Can you work these out from the model? Positions are in its coordinate system, mm. A direction names the side the tool comes from. Coordinates: 2 decimals unless noted, no trailing zeros. Order: outer loops, then holes, each group sorted by start corner. A loop starts at its lowest first (then second) coordinate and runs counter-clockwise, first axis right, second up.
```python
from build123d import *

# Parameters (mm, degrees)
SKETCH1_W           = 22.86
SKETCH1_H           = 20.32
SKETCH1_R           = 1.65
BOSS_EXTRUDE1_DEPTH = 2
SKETCH2_W           = 11.796284554
SKETCH2_H           = 1.966047426
BOSS_EXTRUDE2_DEPTH = 10
SKETCH3_W           = 7.246289084
SKETCH3_H           = 4.830859388
BOSS_EXTRUDE3_DEPTH = 8


with BuildPart() as part:
    # Sketch1 → Boss-Extrude1 (new body)
    with BuildSketch(Plane(origin=(0, 0, 0), x_dir=(1, 0, 0), z_dir=(0, 1, 0))):
        Rectangle(SKETCH1_W, SKETCH1_H)
        with Locations(Location((-8.5, 7.555555556, 0), (0, 0, 270))):
            Circle(SKETCH1_R, mode=Mode.SUBTRACT)
        with Locations(Location((8.5, 7.555555556, 0), (0, 0, 270))):
            Circle(SKETCH1_R, mode=Mode.SUBTRACT)
        with Locations(Location((-8.5, -7.555555556, 0), (0, 0, 270))):
            Circle(SKETCH1_R, mode=Mode.SUBTRACT)
        with Locations(Location((8.5, -7.555555556, 0), (0, 0, 270))):
            Circle(SKETCH1_R, mode=Mode.SUBTRACT)
    extrude(amount=BOSS_EXTRUDE1_DEPTH)

    # Sketch2 → Boss-Extrude2 (add)
    with BuildSketch(Plane.XZ):
        with Locations((0, 7.569282589)):
            Rectangle(SKETCH2_W, SKETCH2_H)
    extrude(amount=BOSS_EXTRUDE2_DEPTH)

    # Sketch3 → Boss-Extrude3 (add)
    with BuildSketch(Plane.XZ):
        with Locations((0, -7.288418671)):
            Rectangle(SKETCH3_W, SKETCH3_H)
    extrude(amount=BOSS_EXTRUDE3_DEPTH)


solid = part.part
```
1. Please list where these lines run through material, in increasing order: probe 1 along Z at (x, y) = (0, -4.5); probe 2 along Y at (x, z) = (9.75, -1.25); probe 3 along Z at (x, y) = (4.5, -2.5).
Completed:
probe 1: z = -9.7 to -4.87, 6.59 to 8.55
probe 2: y = 0 to 2
probe 3: z = 6.59 to 8.55
2. On a 3-axis mill with a long thin cutter (end or side, diameter ignored), from which of +Z, -Z, +X, -X, +Y, -Y can I reach the whole of each face in a straight line? I mean faces 1 (the flat face through (0, -5, 8.552)), 2 (the flat face through (-3.623, -4, -7)), 3 (the flat face through (0, -4, -9.704)), 4 (the flat face through (-5.898, -5, 8)), 5 (the flat face through (0, -5, 6.586)). Say none if no direction works.
Completed:
face 1: +Z, +X, -X, -Y
face 2: -Z, -X, -Y
face 3: -Z, +X, -X, -Y
face 4: +Z, -Z, -X, -Y
face 5: +X, -X, -Y
3. Imagine slicing it at A-A on x = -8.5. Please give me the cut outline in (y, z).
Completed:
outline: (0, -10.16) - (2, -10.16) - (2, -9.21) - (0, -9.21) - close; (0, -5.91) - (2, -5.91) - (2, 5.91) - (0, 5.91) - close; (0, 9.21) - (2, 9.21) - (2, 10.16) - (0, 10.16) - close
4. Thinking about a two-plate mould opening in Z: for faces 6 (the cylindrical face through (7.87, 0.99, 9.08)), 7 (the flat face through (0, 1, 10.16)), 8 (the flat face through (5.898, -5, 8)), which applies, pulls with the +Z half, pulls with the -Z half, needs draft (parallel to the pull), parting line crosses it, or undercut?
Completed:
face 6: undercut
face 7: pulls with the +Z half
face 8: needs draft
5. Imagine slicing it at B-B on y = -2. Please give me the cut outline in (x, z), then the cut area to 3 significant figures.
Completed:
outline: (-5.9, 6.59) - (5.9, 6.59) - (5.9, 8.55) - (-5.9, 8.55) - close; (-3.62, -9.7) - (3.62, -9.7) - (3.62, -4.87) - (-3.62, -4.87) - close
area: 58.2 mm2
6. Imagine slicing it at C-C on y = 1.5. Please give me the cut outline in (x, z), then the cut area to 3 significant figures.
Completed:
outline: (-11.43, -10.16) - (11.43, -10.16) - (11.43, 10.16) - (-11.43, 10.16) - close; hole circle Ø3.3 at (-8.5, -7.56); hole circle Ø3.3 at (-8.5, 7.56); hole circle Ø3.3 at (8.5, -7.56); hole circle Ø3.3 at (8.5, 7.56)
area: 430 mm2
7. I'm going to push flat-ended pins straight in: pin 1 (1.5 mm diameter, centred on x = -6, z = -2, fed in from -Y); pin 2 (1 mm diameter, centred on y = -7, z = 7.5, fed in from +X); pin 3 (4 mm diameter, centred on x = 1, z = -7.5, fed in from -Y). Where does each tip first touch, or does it pass through?
Completed:
pin 1: stops at y = 0
pin 2: stops at x = 5.9
pin 3: stops at y = -8
8. Imagine slicing it at D-D on x = 2.5. Please give me the cut outline in (y, z).
Completed:
outline: (-10, 6.59) - (0, 6.59) - (0, -4.87) - (-8, -4.87) - (-8, -9.7) - (0, -9.7) - (0, -10.16) - (2, -10.16) - (2, 10.16) - (0, 10.16) - (0, 8.55) - (-10, 8.55) - close
